Could you check a few things on this drawing? It's one solid part, dimensions in mm from its lowest x, y, z. A direction names the side the tool comes from. Round coordinates to 2 decimals unless told otherwise and drop trailing zeros. Write each loop counter-clockwise with the first axis right and the second up, starting at its lowest first coordinate (ties: lowest second). Pieces come first, ordered by that corner, then holes. Notation, with made-up numbers: (78.25, -35) - (118.25, -35) arc R25 ccw to (118.25, 3) - close; hole circle Ø3 at (4, 24.5). An arc over 180 degrees is marked (long way). Put each result on its own line as item: value.
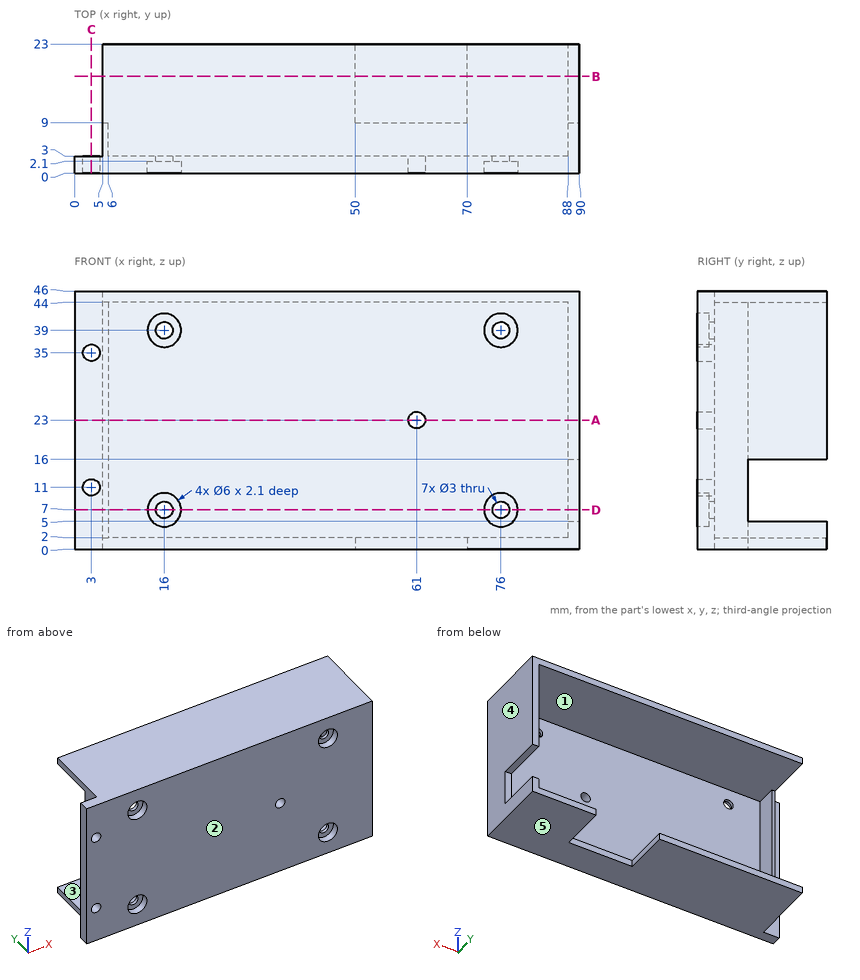
(1) If we mould it in two halves opening along X, with no side actions, what happens to the marked faces 3, 4 and 5? For each: pulls with the +X half, pulls with the -X half, needs draft (parallel to the pull), parting line crosses it, or undercut.
Values found:
face 3: undercut
face 4: pulls with the +X half
face 5: needs draft
(2) Please list where these lines run through material, in increasing order: probe 1 along X at (y, z) = (1, 39); probe 2 along Z at (x, y) = (3, 1.2); probe 3 along Z at (x, y) = (16, 2.7). Write a range as from..to.
Values found:
probe 1: x = 0..13, 19..73, 79..90
probe 2: z = 0..9.5, 12.5..33.5, 36.5..46
probe 3: z = 0..5.5, 8.5..37.5, 40.5..46
(3) I'm going to push flat-ended pins straight in: pin 1 (5 mm diameter, centred on x = 64.5, z = 8, fed in from +Y); pin 2 (2 mm diameter, centred on x = 55, z = 1.5, fed in from +Y); pin 3 (1.8 mm diameter, centred on x = 16, z = 40, fed in from -Y); pin 4 (2.5 mm diameter, centred on x = 16, z = 39, fed in from -Y). Where does each tip first touch, or does it pass through?
Values found:
pin 1: stops at y = 3
pin 2: stops at y = 9
pin 3: stops at y = 2.1
pin 4: passes through
(4) Imagine slicing it at C-C, the plane x = 3. List the corners of the cut face in (y, z) for me.
Values found:
outline: (0, 0) - (3, 0) - (3, 9.5) - (0, 9.5) - close; (0, 12.5) - (3, 12.5) - (3, 33.5) - (0, 33.5) - close; (0, 36.5) - (3, 36.5) - (3, 46) - (0, 46) - close
(5) Imagine slicing it at D-D, the plane z = 7. List the corners of the cut face in (x, y) for me, then the cut area to 3 significant figures.
Values found:
outline: (0, 0) - (13, 0) - (13, 2.1) - (14.5, 2.1) - (14.5, 3) - (6, 3) - (6, 9) - (5, 9) - (5, 3) - (0, 3) - close; (17.5, 2.1) - (19, 2.1) - (19, 0) - (73, 0) - (73, 2.1) - (74.5, 2.1) - (74.5, 3) - (17.5, 3) - close; (77.5, 2.1) - (79, 2.1) - (79, 0) - (90, 0) - (90, 9) - (88, 9) - (88, 3) - (77.5, 3) - close
area: 257 mm^2
(6) Imagine slicing it at B-B, the plane y = 17.25. List the corners of the cut face in (x, z) for me.
Values found:
outline: (5, 0) - (50, 0) - (50, 2) - (5, 2) - close; (5, 44) - (88, 44) - (88, 16) - (90, 16) - (90, 46) - (5, 46) - close; (70, 0) - (90, 0) - (90, 5) - (88, 5) - (88, 2) - (70, 2) - close
(7) Imagine slicing it at A-A, the plane z = 23. List the corners of the cut face in (x, y) for me, then the cut area to 3 significant figures.
Values found:
outline: (0, 0) - (59.5, 0) - (59.5, 3) - (6, 3) - (6, 9) - (5, 9) - (5, 3) - (0, 3) - close; (62.5, 0) - (90, 0) - (90, 23) - (88, 23) - (88, 3) - (62.5, 3) - close
area: 307 mm^2
(8) For the marked faces 1 and 2, which set-ups out of +Z, -Z, +X, -X, +Y, -Y let a thin tool reach every point of the face, with its end or its side?
Values found:
face 1: +Y
face 2: +Z, -Z, +X, -X, -Y
